Input: dimensioned drawing with shaded views. Units: mm. Origin: part minimum x, y, z. Coordinates: 2 decimals unless noted, no trailing zeros. Order: outer loops, then holes, each group sorted by start corner. A loop starts at its lowest first (then second) coordinate and runs counter-clockwise, first axis right, second up. Notation, with made-up numbers: M 61,76 L 96,76 A20 cw 96,90 Z; hole C 54,58.25 d4. An arc over 180 degrees is marked long. Use CSV: the item, a comma, the result in double quotes. Start each with the question number.
1. First-contact query: P1, Ø11.5, axis at x = 34.5, z = 68, coming from the -Y side; P2, Ø10, axis at y = 29, z = 34.5, coming from the +X side; P3, Ø4, axis at y = 43.5, z = 31.5, coming from the +X side. Flat tips, straight axial feed; report the tip coordinate or a pass-through.
2. Material intervals for line 1 (Y direction, x = 30, z = 25); line 2 (X direction, y = 44.5, z = 55); line 3 (Y direction, x = 14.5, z = 50), sorted ascending.
3. Section query A-A on y = 30. Return the cut outline in (x, z), and give its area (3 significant figures).
4. Pull-direction query (X, two-part tool) for the marked faces 1, 2, 3 and 4; classes: pulls with the +X half, pulls with the -X half, needs draft (parallel to the pull), parting line crosses it, or undercut.
5. Section query D-D on y = 56. Return the cut outline in (x, z).
6. Section query C-C on z = 78. Return the cut outline in (x, y).
7. Section query B-B on x = 30. Return the cut outline in (y, z).
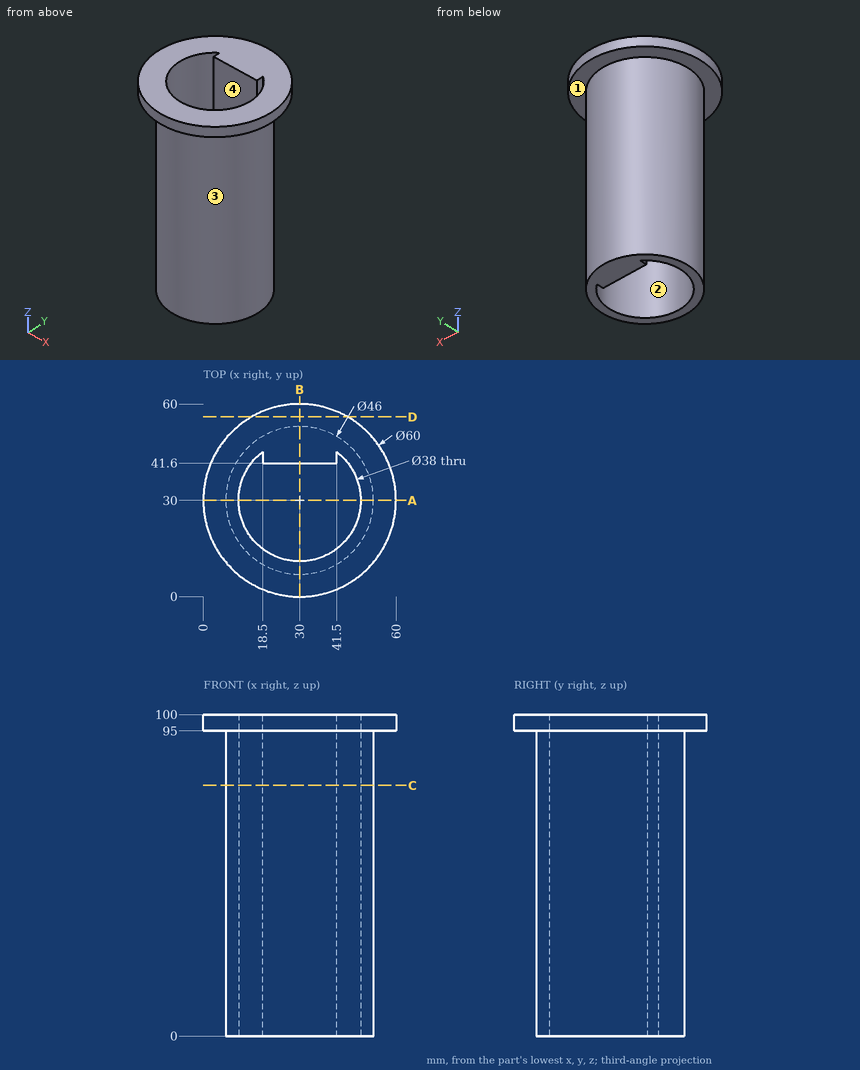
Results list:
1,P1,"stops at y = 7"
1,P2,"stops at x = 53"
1,P3,"stops at x = 49.92"
2,line 1,"y = 7 to 11, 41.6 to 53"
2,line 2,"x = 12.15 to 17.72, 18.5 to 41.5, 42.28 to 47.85"
2,line 3,"y = 13.01 to 19.01, 40.99 to 46.99"
3,outline,"M 0,95 L 7,95 L 7,0 L 11,0 L 11,100 L 0,100 Z; M 49,0 L 53,0 L 53,95 L 60,95 L 60,100 L 49,100 Z"
3,area,"870 mm²"
4,face 1,"needs draft"
4,face 2,"undercut"
4,face 3,"parting line crosses it"
4,face 4,"undercut"
5,outline,"M 15.03,95 L 44.97,95 L 44.97,100 L 15.03,100 Z"
6,outline,"C 30,30 d46; hole M 18.5,41.6 L 18.5,45.12 A19 ccw long 41.5,45.12 L 41.5,41.6 Z"
7,outline,"M 0,95 L 7,95 L 7,0 L 11,0 L 11,100 L 0,100 Z; M 41.6,0 L 53,0 L 53,95 L 60,95 L 60,100 L 41.6,100 Z"
